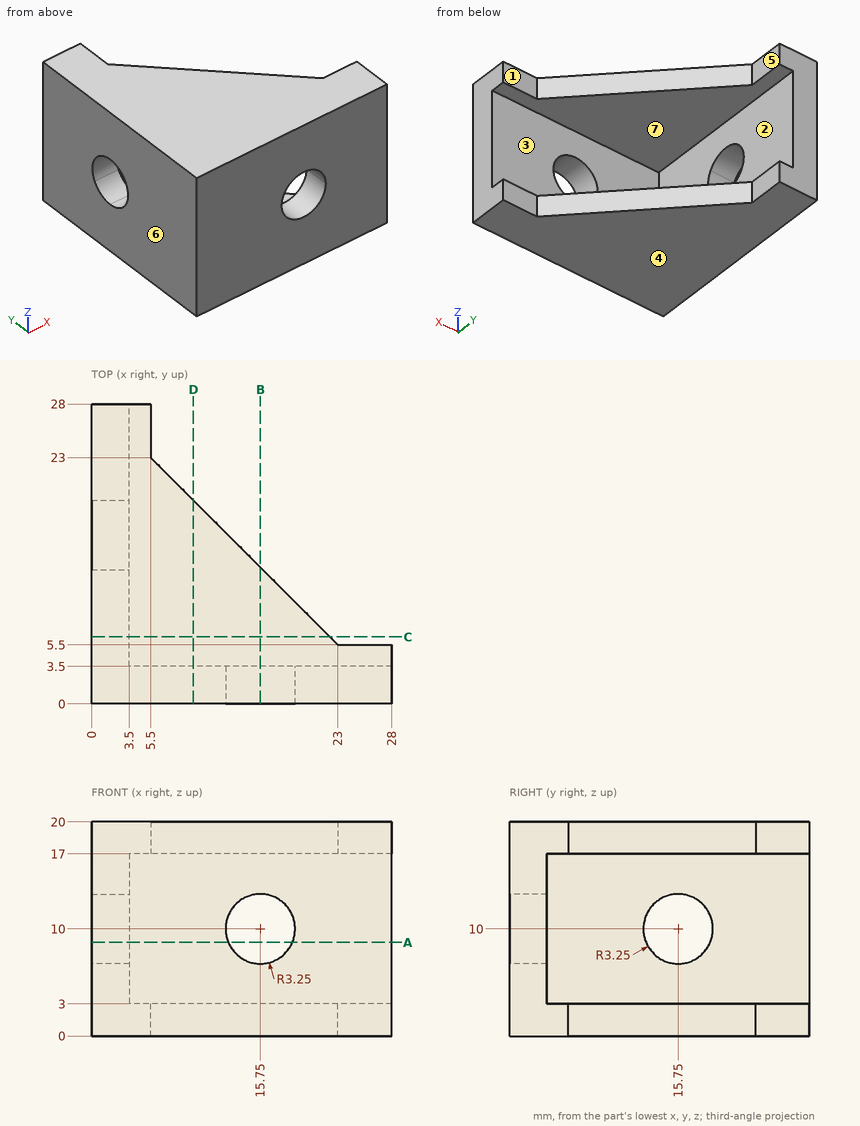
For this review, use the dimensioned drawing (mm, ordinates from the lowest corner) and the shaded views. A direction names the side the tool comes from. Give positions to 0.01 mm unless a question says otherwise; leave off trailing zeros. Write each loop counter-clockwise with the first axis right and the second up, starting at its lowest first coordinate (ties: lowest second). Pieces come first, ordered by that corner, then holes. Notation, with made-up numbers: M 17.25,-20.5 L 49.25,-20.5 A22 cw 49.25,12.5 Z; hole C 46.5,26.5 d2. An arc over 180 degrees is marked long. Answer as a JSON object with one key per item and string values. Group by question number.
Item 1: Consider section C-C on y = 6.25. Write out the cut boundary in (x, z).
Item 2: Consider section B-B on x = 15.75. Write out the cut boundary in (y, z).
Item 3: For probe 1 along Z at (x, y) = (5.25, 11); probe 2 along X at (y, z) = (22.5, 3.5), list the stretches that pass through material, from the lowest coordinate up. Write a range as [from, to].
Item 4: Tool access review of the marked faces 5, 6 and 7: name each direction out of +Z, -Z, +X, -X, +Y, -Y from which nothing blocks a thin tool from reaching the whole face with its end or side.
Item 5: Consider section D-D on x = 9.5. Write out the cut boundary in (y, z), plus the area to 3 significant figures.
Item 6: Consider section A-A on z = 8.75. Write out the cut boundary in (x, y).
Item 7: Draft analysis for pull direction Z (two halves, no side actions). For the marked faces 1, 2, 3 and 4, state which applies: +Z half, -Z half, draft (parallel to the pull), parting line (faces both ways), or undercut.
Item 8: For pin 1 Ø1 at (y, z) = (10, 8.5) entering from +X; pin 2 Ø1.5 at (x, z) = (22, 8) entering from +Y; pin 3 Ø1 at (x, z) = (14.5, 12) entering from +Y; pin 4 Ø1.5 at (y, z) = (26, 19) entering from +X, all flat-tipped, find the tip position at first contact; note any pin that passes through.
Check result:
{
 "1": {"outline": "M 0,0 L 22.25,0 L 22.25,3 L 3.5,3 L 3.5,17 L 22.25,17 L 22.25,20 L 0,20 Z"},
 "2": {"outline": "M 0,0 L 12.75,0 L 12.75,3 L 3.5,3 L 3.5,6.75 L 0,6.75 Z; M 0,13.25 L 3.5,13.25 L 3.5,17 L 12.75,17 L 12.75,20 L 0,20 Z"},
 "3": {"probe 1": "z = [0, 3], [17, 20]", "probe 2": "x = [0, 3.5]"},
 "4": {"face 5": "+Z, -Z, +X, +Y", "face 6": "+Z, -Z, -X, +Y, -Y", "face 7": "+X, +Y"},
 "5": {"outline": "M 0,0 L 19,0 L 19,3 L 3.5,3 L 3.5,17 L 19,17 L 19,20 L 0,20 Z", "area": "163 mm^2"},
 "6": {"outline": "M 0,0 L 12.75,0 L 12.75,3.5 L 3.5,3.5 L 3.5,12.75 L 0,12.75 Z; M 0,18.75 L 3.5,18.75 L 3.5,28 L 0,28 Z; M 18.75,0 L 28,0 L 28,3.5 L 18.75,3.5 Z"},
 "7": {"face 1": "draft", "face 2": "undercut", "face 3": "undercut", "face 4": "-Z half"},
 "8": {"pin 1": "stops at x = 3.5", "pin 2": "stops at y = 3.5", "pin 3": "passes through", "pin 4": "stops at x = 5.5"}
}
